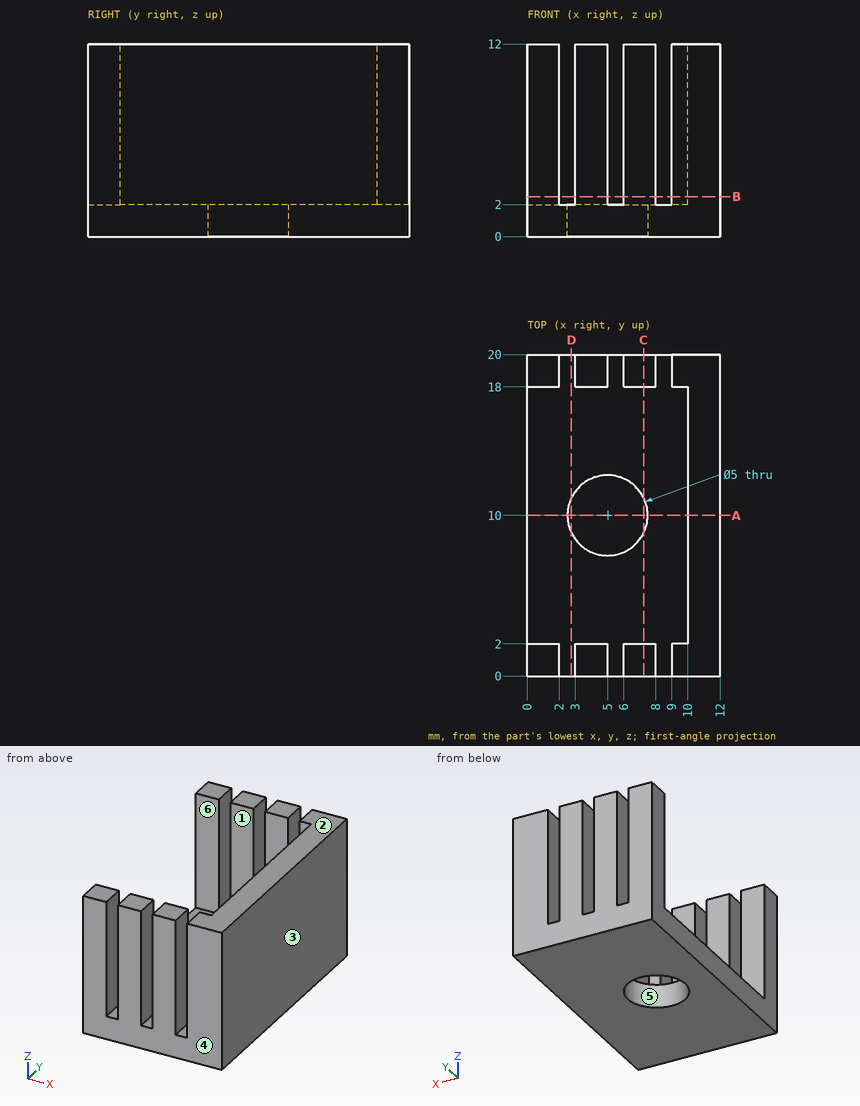
Print and shaded views of the part. All mm, measured from the part's lowest x, y and z. A direction names the side the tool comes from. Round coordinates to 2 decimals unless told otherwise and drop trailing zeros. Write each loop counter-clockwise with the first axis right and the second up, starting at its lowest first coordinate (ties: lowest second). Pieces come first, ordered by that corner, then holes. Notation, with made-up numbers: (73, 30.25) - (99, 30.25) arc R8 cw to (99, 34.25) - close; hole circle Ø2 at (-31.5, 21). An arc over 180 degrees is marked (long way). One line per item, written item: value.
(1) Wall check: probe 1 along X at (y, z) = (1.75, 9.75); probe 2 along Y at (x, z) = (5, 1.1); probe 3 along Y at (x, z) = (3.25, 7.75). Give the ranges that are in metal, low to high.
Values follow:
probe 1: x = 0 to 2, 3 to 5, 6 to 8, 9 to 12
probe 2: y = 0 to 7.5, 12.5 to 20
probe 3: y = 0 to 2, 18 to 20
(2) Cut at B-B, the plane z = 2.5. Give the number of separate pieces and of enclosed holes in the cut face, plus the area to 3 significant figures.
Values follow:
separate pieces: 7
enclosed holes: 0
area: 68.0 mm²
(3) Two-plate mould, pull along Y, no slides. Class the marked faces 3, 4, 5 and 6: pulls with the +Y half, pulls with the -Y half, needs draft (parallel to the pull), parting line crosses it, or undercut.
Values follow:
face 3: needs draft
face 4: pulls with the -Y half
face 5: undercut
face 6: undercut
(4) Drop flat-ended pins along their axis: P1, Ø1.5, axis at y = 4, z = 3.5, coming from the -X side; P2, Ø3, axis at x = 3.5, y = 6.5, coming from the +Z side. Give the stop position or say it passes through.
Values follow:
P1: stops at x = 10
P2: stops at z = 2
(5) 3-axis set-ups, long thin cutter, end or side, ignore diameter. For the marked faces 1 and 2: which of +Z, -Z, +X, -X, +Y, -Y reach the whole face in a straight line?
Values follow:
face 1: +Z, -X
face 2: +Z, +X, -X, +Y, -Y
(6) Cut at D-D, the plane x = 2.75. Give the cut face in (y, z).
Values follow:
outline: (0, 0) - (8.91, 0) - (8.91, 2) - (0, 2) - close; (11.09, 0) - (20, 0) - (20, 2) - (11.09, 2) - close
(7) Cut at A-A, the plane y = 10. Give the cut face in (x, z), plus the area to 3 significant figures.
Values follow:
outline: (0, 0) - (2.5, 0) - (2.5, 2) - (0, 2) - close; (7.5, 0) - (12, 0) - (12, 12) - (10, 12) - (10, 2) - (7.5, 2) - close
area: 34.0 mm²
(8) Cut at C-C, the plane x = 7.25. Give the cut face in (y, z).
Values follow:
outline: (0, 0) - (8.91, 0) - (8.91, 2) - (2, 2) - (2, 12) - (0, 12) - close; (11.09, 0) - (20, 0) - (20, 12) - (18, 12) - (18, 2) - (11.09, 2) - close
